Here's how the part is built. I have some questions about the finished solid (model axes, mm). Round coordinates to 2 decimals unless told otherwise and drop trailing zeros. Loops run counter-clockwise (first coordinate to the right, second up) from the corner with the lowest first, then second, coordinate; pieces in that order, holes last. Notation, with made-up numbers: M -17.75,3.25 L 34.25,3.25 A10 ccw 34.25,17.25 Z; hole C 11,58.5 d9. An arc over 180 degrees is marked long. Use a Markdown table: item, result.
from build123d import *

# Parameters (mm, degrees)
F0_W     = 1000
F0_H     = 700
F1_DEPTH = 400
F2_R     = 300
F3_R     = 99.99999


# Not quite as in the source:
# - a fillet or chamfer is up to 0.001 mm smaller than in the source, because OpenCascade refuses the exact size


with BuildPart() as f1:
    # F0 (on Top) → F1 (new body)
    with BuildSketch(Plane.XY):
        Rectangle(F0_W, F0_H)
    extrude(amount=F1_DEPTH)

    # F2
    f2_edges = [f1.edges().sort_by_distance(p)[0] for p in [
        (0, -350, 400),
        (0, 350, 400),
    ]]
    fillet(f2_edges, radius=F2_R)

    # F3 (radius 100 in the source; OpenCascade refuses exactly that, so slightly less here)
    f3_edges = [f1.edges().sort_by_distance(p)[0] for p in [
        (0, 350, 0),
        (0, -350, 0),
    ]]
    fillet(f3_edges, radius=F3_R)


solid = f1.part
1. Imagine slicing it at B-B, the plane y = 148. Write out the boundary of the cut face in (x, z), then the cut area to 3 significant figures.
Answer sheet:
| item | result |
|---|---|
| outline | M -500,0 L 500,0 L 500,383.54 L -500,383.54 Z |
| area | 384,000 mm2 |
2. I need wall thicknesses on probe 1 along Y at (x, z) = (-208.5, 102.5); probe 2 along Z at (x, y) = (-171.5, 170); probe 3 along Z at (x, y) = (117, -103.5). Which ranges of each line are inside material? Lowest first, please. Write a range as from..to.
Answer sheet:
| item | result |
|---|---|
| probe 1 | -349.99..349.99 |
| probe 2 | 0..374.95 |
| probe 3 | 0..395.19 |
3. For pin 1 Ø1.5 at (x, z) = (67, 272.5) entering from -Y; pin 2 Ø10 at (x, z) = (-195.5, 305.5) entering from +Y; pin 3 Ø1 at (x, z) = (134, 295.5) entering from +Y, each with a flat end and sliding along its axis, tell me the tip position at first contact or that it passes through.
Answer sheet:
| item | result |
|---|---|
| pin 1 | y = -295.97 |
| pin 2 | y = 273.16 |
| pin 3 | y = 277.98 |
4. Imagine slicing it at C-C, the plane z = 372.5. Write out the boundary of the cut face in (x, y), then the cut area to 3 significant figures.
Answer sheet:
| item | result |
|---|---|
| outline | M -500,-175.47 L 500,-175.47 L 500,175.47 L -500,175.47 Z |
| area | 351,000 mm2 |
